```python
from build123d import *

# Parameters (mm, degrees)
SKETCH2_R           = 10
BOSS_EXTRUDE1_DEPTH = 135
SKETCH3_R           = 10
SKETCH3_R_2         = 9.43
CUT_EXTRUDE2_DEPTH  = 1.1
SKETCH4_W           = 6
SKETCH4_H           = 3.067792635
CUT_EXTRUDE3_DEPTH  = 61.25
SKETCH5_R           = 11
BOSS_EXTRUDE2_DEPTH = 70
FILLET3_R           = 2
SKETCH6_R           = 11
SKETCH6_R_2         = 10.35
CUT_EXTRUDE4_DEPTH  = 1.1
CUT_EXTRUDE5_DEPTH  = 2.5


with BuildPart() as part:
    # Sketch2 → Boss-Extrude1 (new body)
    with BuildSketch(Plane.XY):
        Circle(SKETCH2_R)
    extrude(amount=BOSS_EXTRUDE1_DEPTH)

    # Sketch3 → Cut-Extrude2 (cut)
    with BuildSketch(Plane(origin=(0, 0, 5), x_dir=(-1, 0, 0), z_dir=(0, 0, -1))):
        Circle(SKETCH3_R)
        Circle(SKETCH3_R_2, mode=Mode.SUBTRACT)
    cut_extrude2 = extrude(amount=-CUT_EXTRUDE2_DEPTH, mode=Mode.SUBTRACT)

    # Mirror1: Cut-Extrude2 across plane
    add(cut_extrude2.mirror(Plane(origin=(0, 0, 67.35), x_dir=(1, 0, 0), z_dir=(0, 0, -1))), mode=Mode.SUBTRACT)

    # Sketch4 → Cut-Extrude3 (cut, symmetric)
    with BuildSketch(Plane(origin=(0, 0, 67.35), x_dir=(-1, 0, 0), z_dir=(0, 0, -1))):
        with Locations((0, 9.343896318)):
            Rectangle(SKETCH4_W, SKETCH4_H)
    extrude(amount=CUT_EXTRUDE3_DEPTH, both=True, mode=Mode.SUBTRACT)

    # Sketch5 → Boss-Extrude2 (add)
    with BuildSketch(Plane.XY.offset(135)):
        Circle(SKETCH5_R)
    extrude(amount=BOSS_EXTRUDE2_DEPTH)

    # Fillet3
    # the kernel refuses this fillet: 2 mm, written as the material it adds along each edge
    with BuildSketch(Plane(origin=(0, 0, 135), x_dir=(1, 0, 0), z_dir=(0, -1, 0))) as fillet3_piece_1:
        with BuildLine():
            CenterArc((12, -1.732050808), FILLET3_R, 120, 60)
            Line((10, -1.732050808), (9.96, -1.732050808))
            Line((9.96, -1.732050808), (9.96, 0))
            Line((9.96, 0), (10, 0.04))
            ThreePointArc((10, 0.04), (10.5, 0.04), (10.98, 0.034641016))
            Line((10.98, 0.034641016), (11, 0))
        make_face()
    revolve(axis=Axis((0, 0, 135), (0, 0, 1)))

    # Sketch6 → Cut-Extrude4 (cut)
    with BuildSketch(Plane.XY.offset(135)):
        Circle(SKETCH6_R)
        Circle(SKETCH6_R_2, mode=Mode.SUBTRACT)
    cut_extrude4 = extrude(amount=CUT_EXTRUDE4_DEPTH, mode=Mode.SUBTRACT)

    # Mirror2: Cut-Extrude4 across plane
    add(cut_extrude4.mirror(Plane.XY.offset(166.1)), mode=Mode.SUBTRACT)

    # Sketch8 → Cut-Extrude5 (cut)
    with BuildSketch(Plane(origin=(0, 11, 0), x_dir=(1, 0, 0), z_dir=(0, 1, 0))):
        with BuildLine():
            Line((3, -146.1), (3, -186.1))
            ThreePointArc((3, -186.1), (0, -189.1), (-3, -186.1))
            Line((-3, -186.1), (-3, -146.1))
            ThreePointArc((-3, -146.1), (0, -143.1), (3, -146.1))
        make_face()
    extrude(amount=-CUT_EXTRUDE5_DEPTH, mode=Mode.SUBTRACT)


solid = part.part
```
Part model, mm, in its own coordinate system. A direction names the side the tool comes from. Round coordinates to 2 decimals unless told otherwise and drop trailing zeros. Order: outer loops, then holes, each group sorted by start corner. A loop starts at its lowest first (then second) coordinate and runs counter-clockwise, first axis right, second up. Notation, with made-up numbers: M -24,19 L 7,19 A13 cw 7,34 Z; hole C -4.75,-34.75 d6. An arc over 180 degrees is marked long. Put each result on its own line as item: value. Start each with the question number.
1. Two-plate mould, pull along Z, no slides. Class faces 1 (the face through (1.23, 9.35, 5.54)), 2 (the face through (-2.38, -10.74, 201.05)), 3 (the face through (0, 0, 0)): +Z half, -Z half, draft (parallel to the pull), parting line (faces both ways), or undercut.
2. Drop flat-ended pins along their axis: pin 1 (1.4 mm diameter, centred on y = 8.5, z = 44, fed in from -X); pin 2 (1.9 mm diameter, centred on y = 8.5, z = 37, fed in from +X); pin 3 (4 mm diameter, centred on x = -5.5, z = 137.5, fed in from -Y). Give the stop position or say it passes through.
3. Slice it at B-B on z = 96. List the corners of the cut face in (x, y), then the cut area to 3 significant figures.
4. Tool access for faces 4 (the face through (-4, -9, 6.1)), 5 (the face through (-2.17, -9.76, 2.46)), 6 (the face through (0, 7.81, 66)): list every direction of +Z, -Z, +X, -X, +Y, -Y with a clear straight run to the whole face (end or side of a thin tool).
5. Slice it at A-A on z = 181.5. List the corners of the cut face in (x, y), then the cut area to 3 significant figures.
6. Drill centre lines: probe 1 along X at (y, z) = (8.5, 12); probe 2 along X at (y, z) = (0.5, 169); probe 3 along Y at (x, z) = (-0.25, 175.5). Where is each one in solid material? Low to high. Write a range as [from, to].
Findings:
1. face 1: undercut
1. face 2: draft
1. face 3: -Z half
2. pin 1: x = -6.26
2. pin 2: x = 6.56
2. pin 3: y = -10.43
3. outline: M -3,7.81 L -3,9.54 A10 ccw long 3,9.54 L 3,7.81 Z
3. area: 302 mm2
4. face 4: none
4. face 5: -Z
4. face 6: +Y
5. outline: M -3,8.5 L -3,10.58 A11 ccw long 3,10.58 L 3,8.5 Z
5. area: 366 mm2
6. probe 1: [-5.27, -3], [3, 5.27]
6. probe 2: [-10.99, 10.99]
6. probe 3: [-11, 8.5]
